Read the model definition and answer for the solid it produces. Units are mm, in the model's axes. A direction names the side the tool comes from. Coordinates: 2 decimals unless noted, no trailing zeros. Loops run counter-clockwise (first coordinate to the right, second up) from the corner with the lowest first, then second, coordinate; pieces in that order, holes last.
from build123d import *

# Parameters (mm, degrees)
F0_W     = 184.15
F0_H     = 101.6
F1_DEPTH = 3
F3_W     = 8
F3_H     = 25
F3_R     = 1.5
F2_R     = 1.5
F2_R_2   = 2.25
F4_DEPTH = 3.001
F5_W     = 12.7
F5_H     = 12.7
F6_DEPTH = 5
F7_R     = 1.5
F8_DEPTH = 8.001


with BuildPart() as f1:
    # F0 (on Top) → F1 (new body)
    with BuildSketch(Plane.XY):
        with Locations((3.175, 0)):
            Rectangle(F0_W, F0_H)
    extrude(amount=F1_DEPTH)

    # F3 (on face) + F2 (on Top) → F4 (cut, through all)
    with BuildSketch(Plane.XY.offset(3)):
        with Locations((75.875, 31.55)):
            Rectangle(F3_W, F3_H)
        with Locations((-75.875, 0)):
            Rectangle(F3_W, F3_H)
        with Locations((75.875, -31.55)):
            Rectangle(F3_W, F3_H)
        with Locations((-67.875, 0)):
            Circle(F3_R)
        with Locations((-83.875, 0)):
            Circle(F3_R)
        with Locations((83.875, 31.55)):
            Circle(F3_R)
        with Locations((67.875, 31.55)):
            Circle(F3_R)
        with Locations((83.875, -31.55)):
            Circle(F3_R)
        with Locations((67.875, -31.55)):
            Circle(F3_R)
        with Locations((0.03105, 20.5)):
            Circle(F3_R)
        with Locations((0, -20.5)):
            Circle(F3_R)
    with BuildSketch(Plane.XY):
        with BuildLine():
            Line((103.423341, 112.311256), (-105.576659, 112.311256))
            ThreePointArc((-105.576659, 112.311256), (-110.87996, 110.114557), (-113.076659, 104.811256))
            Line((-113.076659, 104.811256), (-113.076659, -104.188744))
            ThreePointArc((-113.076659, -104.188744), (-110.87996, -109.492044), (-105.576659, -111.688744))
            Line((-105.576659, -111.688744), (103.423341, -111.688744))
            ThreePointArc((103.423341, -111.688744), (108.726642, -109.492044), (110.923341, -104.188744))
            Line((110.923341, -104.188744), (110.923341, 104.811256))
            ThreePointArc((110.923341, 104.811256), (108.726642, 110.114557), (103.423341, 112.311256))
        make_face()
        with Locations((-105.576659, -104.188744)):
            Circle(F2_R, mode=Mode.SUBTRACT)
        with BuildLine():
            Line((-73.691883, -86.446103), (-28.691883, -41.446103))
            ThreePointArc((-28.691883, -41.446103), (-26.745343, -40.145466), (-24.449242, -39.688744))
            Line((-24.449242, -39.688744), (-12.076659, -39.688744))
            ThreePointArc((-12.076659, -39.688744), (-7.834019, -41.446103), (-6.076659, -45.688744))
            Line((-6.076659, -45.688744), (-6.076659, -90.688744))
            ThreePointArc((-6.076659, -90.688744), (-7.834019, -94.931384), (-12.076659, -96.688744))
            Line((-12.076659, -96.688744), (-69.449242, -96.688744))
            ThreePointArc((-69.449242, -96.688744), (-74.992519, -92.984844), (-73.691883, -86.446103))
        make_face(mode=Mode.SUBTRACT)
        with Locations((-98.576659, -39.688744)):
            Circle(F2_R_2, mode=Mode.SUBTRACT)
        with BuildLine():
            Line((-90.676659, -24.688744), (-86.476659, -24.688744))
            ThreePointArc((-86.476659, -24.688744), (-84.355339, -25.567423), (-83.476659, -27.688744))
            Line((-83.476659, -27.688744), (-83.476659, -51.688744))
            ThreePointArc((-83.476659, -51.688744), (-84.355339, -53.810064), (-86.476659, -54.688744))
            Line((-86.476659, -54.688744), (-90.676659, -54.688744))
            ThreePointArc((-90.676659, -54.688744), (-92.79798, -53.810064), (-93.676659, -51.688744))
            Line((-93.676659, -51.688744), (-93.676659, -27.688744))
            ThreePointArc((-93.676659, -27.688744), (-92.79798, -25.567423), (-90.676659, -24.688744))
        make_face(mode=Mode.SUBTRACT)
        with Locations((-78.576659, -39.688744)):
            Circle(F2_R_2, mode=Mode.SUBTRACT)
        with BuildLine():
            ThreePointArc((22.295924, -39.688744), (24.592024, -40.145466), (26.538564, -41.446103))
            Line((26.538564, -41.446103), (71.538564, -86.446103))
            ThreePointArc((71.538564, -86.446103), (72.839201, -92.984844), (67.295924, -96.688744))
            Line((67.295924, -96.688744), (9.923341, -96.688744))
            ThreePointArc((9.923341, -96.688744), (5.6807, -94.931384), (3.923341, -90.688744))
            Line((3.923341, -90.688744), (3.923341, -45.688744))
            ThreePointArc((3.923341, -45.688744), (5.6807, -41.446103), (9.923341, -39.688744))
            Line((9.923341, -39.688744), (22.295924, -39.688744))
        make_face(mode=Mode.SUBTRACT)
        with Locations((103.423341, -104.188744)):
            Circle(F2_R, mode=Mode.SUBTRACT)
        with Locations((-1.076659, -20.188744)):
            Circle(F2_R, mode=Mode.SUBTRACT)
        with BuildLine():
            ThreePointArc((95.923341, -68.061327), (92.219441, -73.604604), (85.6807, -72.303967))
            Line((85.6807, -72.303967), (49.165981, -35.789249))
            ThreePointArc((49.165981, -35.789249), (47.865345, -29.250507), (53.408622, -25.546608))
            Line((53.408622, -25.546608), (89.923341, -25.546608))
            ThreePointArc((89.923341, -25.546608), (94.165981, -27.303967), (95.923341, -31.546608))
            Line((95.923341, -31.546608), (95.923341, -68.061327))
        make_face(mode=Mode.SUBTRACT)
        with BuildLine():
            Line((84.323341, 15.311256), (88.523341, 15.311256))
            ThreePointArc((88.523341, 15.311256), (90.644661, 14.432577), (91.523341, 12.311256))
            Line((91.523341, 12.311256), (91.523341, -11.688744))
            ThreePointArc((91.523341, -11.688744), (90.644661, -13.810064), (88.523341, -14.688744))
            Line((88.523341, -14.688744), (84.323341, -14.688744))
            ThreePointArc((84.323341, -14.688744), (82.20202, -13.810064), (81.323341, -11.688744))
            Line((81.323341, -11.688744), (81.323341, 12.311256))
            ThreePointArc((81.323341, 12.311256), (82.20202, 14.432577), (84.323341, 15.311256))
        make_face(mode=Mode.SUBTRACT)
        with Locations((-98.576659, 40.311256)):
            Circle(F2_R_2, mode=Mode.SUBTRACT)
        with BuildLine():
            ThreePointArc((-83.476659, 28.311256), (-84.355339, 26.189936), (-86.476659, 25.311256))
            Line((-86.476659, 25.311256), (-90.676659, 25.311256))
            ThreePointArc((-90.676659, 25.311256), (-92.79798, 26.189936), (-93.676659, 28.311256))
            Line((-93.676659, 28.311256), (-93.676659, 52.311256))
            ThreePointArc((-93.676659, 52.311256), (-92.79798, 54.432577), (-90.676659, 55.311256))
            Line((-90.676659, 55.311256), (-86.476659, 55.311256))
            ThreePointArc((-86.476659, 55.311256), (-84.355339, 54.432577), (-83.476659, 52.311256))
            Line((-83.476659, 52.311256), (-83.476659, 28.311256))
        make_face(mode=Mode.SUBTRACT)
        with Locations((-78.576659, 40.311256)):
            Circle(F2_R_2, mode=Mode.SUBTRACT)
        with Locations((-105.576659, 104.811256)):
            Circle(F2_R, mode=Mode.SUBTRACT)
        with BuildLine():
            ThreePointArc((-12.076659, 97.311256), (-7.834019, 95.553897), (-6.076659, 91.311256))
            Line((-6.076659, 91.311256), (-6.076659, 46.311256))
            ThreePointArc((-6.076659, 46.311256), (-7.834019, 42.068616), (-12.076659, 40.311256))
            Line((-12.076659, 40.311256), (-24.449242, 40.311256))
            ThreePointArc((-24.449242, 40.311256), (-26.745343, 40.767979), (-28.691883, 42.068616))
            Line((-28.691883, 42.068616), (-73.691883, 87.068616))
            ThreePointArc((-73.691883, 87.068616), (-74.992519, 93.607357), (-69.449242, 97.311256))
            Line((-69.449242, 97.311256), (-12.076659, 97.311256))
        make_face(mode=Mode.SUBTRACT)
        with Locations((-1.076659, 20.811256)):
            Circle(F2_R, mode=Mode.SUBTRACT)
        with Locations((76.423341, 0.311256)):
            Circle(F2_R_2, mode=Mode.SUBTRACT)
        with Locations((96.423341, 0.311256)):
            Circle(F2_R_2, mode=Mode.SUBTRACT)
        with BuildLine():
            ThreePointArc((53.408622, 26.169121), (47.865345, 29.87302), (49.165981, 36.411762))
            Line((49.165981, 36.411762), (85.6807, 72.92648))
            ThreePointArc((85.6807, 72.92648), (92.219441, 74.227117), (95.923341, 68.683839))
            Line((95.923341, 68.683839), (95.923341, 32.169121))
            ThreePointArc((95.923341, 32.169121), (94.165981, 27.92648), (89.923341, 26.169121))
            Line((89.923341, 26.169121), (53.408622, 26.169121))
        make_face(mode=Mode.SUBTRACT)
        with BuildLine():
            Line((3.923341, 46.311256), (3.923341, 91.311256))
            ThreePointArc((3.923341, 91.311256), (5.6807, 95.553897), (9.923341, 97.311256))
            Line((9.923341, 97.311256), (67.295924, 97.311256))
            ThreePointArc((67.295924, 97.311256), (72.839201, 93.607357), (71.538564, 87.068616))
            Line((71.538564, 87.068616), (26.538564, 42.068616))
            ThreePointArc((26.538564, 42.068616), (24.592024, 40.767979), (22.295924, 40.311256))
            Line((22.295924, 40.311256), (9.923341, 40.311256))
            ThreePointArc((9.923341, 40.311256), (5.6807, 42.068616), (3.923341, 46.311256))
        make_face(mode=Mode.SUBTRACT)
        with Locations((103.423341, 104.811256)):
            Circle(F2_R, mode=Mode.SUBTRACT)
    extrude(amount=-F4_DEPTH, mode=Mode.SUBTRACT)

    # F5 (on face) → F6 (join)
    with BuildSketch(Plane.XY.offset(3)):
        with Locations((88.9, -44.45)):
            Rectangle(F5_W, F5_H)
        with Locations((-82.55, -44.45)):
            Rectangle(F5_W, F5_H)
        with Locations((-82.55, 44.45)):
            Rectangle(F5_W, F5_H)
        with Locations((88.9, 44.45)):
            Rectangle(F5_W, F5_H)
    extrude(amount=F6_DEPTH)

    # F7 (on face) → F8 (cut, through all)
    with BuildSketch(Plane.XY.offset(8)):
        with Locations((-82.55, 44.45)):
            Circle(F7_R)
        with Locations((88.9, 44.45)):
            Circle(F7_R)
        with Locations((88.9, -44.45)):
            Circle(F7_R)
        with Locations((-82.55, -44.45)):
            Circle(F7_R)
    extrude(amount=-F8_DEPTH, mode=Mode.SUBTRACT)


solid = f1.part
Item 1: A cutting plane is placed at B-B on y = -17. Determine the outline of the cut face in (x, z).
Numbers:
outline: (-88.9, 0) - (95.25, 0) - (95.25, 3) - (-88.9, 3) - close
Item 2: Which of the six approach directions +Z, -Z, +X, -X, +Y, -Y give full straight-line access (tool end or side, diameter ignored) to faces 1 (the face through (89, -38.1, 5)), 2 (the face through (-84, -43, 8)), 3 (the face through (82.55, 44, 5))?
Numbers:
face 1: +Z, +X, -X
face 2: +Z, +X, -X, +Y, -Y
face 3: +Z, +Y, -Y
Item 3: A cutting plane is placed at A-A on x = 64.5. Determine the outline of the cut face in (y, z).
Numbers:
outline: (-50.8, 0) - (50.8, 0) - (50.8, 3) - (-50.8, 3) - close
Item 4: Determine the mould class of faces 4 (the face through (89, 38.1, 5)), 5 (the face through (-88.9, -1, 2)), 6 (the face through (82.55, -45, 5)) for opening direction X: released by +X, released by -X, zero draft, split by the parting line, or undercut.
Numbers:
face 4: zero draft
face 5: released by -X
face 6: undercut
Item 5: Given pin 1 (5 mm diameter, centred on x = -35, y = 15, fed in from -Z), flat-ended and moving along its own axis, determine where the tip first touches the part or whether it passes through.
Numbers:
pin 1: stops at z = 0
Item 6: Find the intervals of material crossed by line 1 along Y through (x, z) = (88.9, 5); line 2 along Y through (x, z) = (75, 2.25); line 3 along Y through (x, z) = (83, 4.25), in increasing order.
Numbers:
line 1: y = -50.8 to -45.95, -42.95 to -38.1, 38.1 to 42.95, 45.95 to 50.8
line 2: y = -50.8 to -44.05, -19.05 to 19.05, 44.05 to 50.8
line 3: y = -50.8 to -38.1, 38.1 to 50.8
